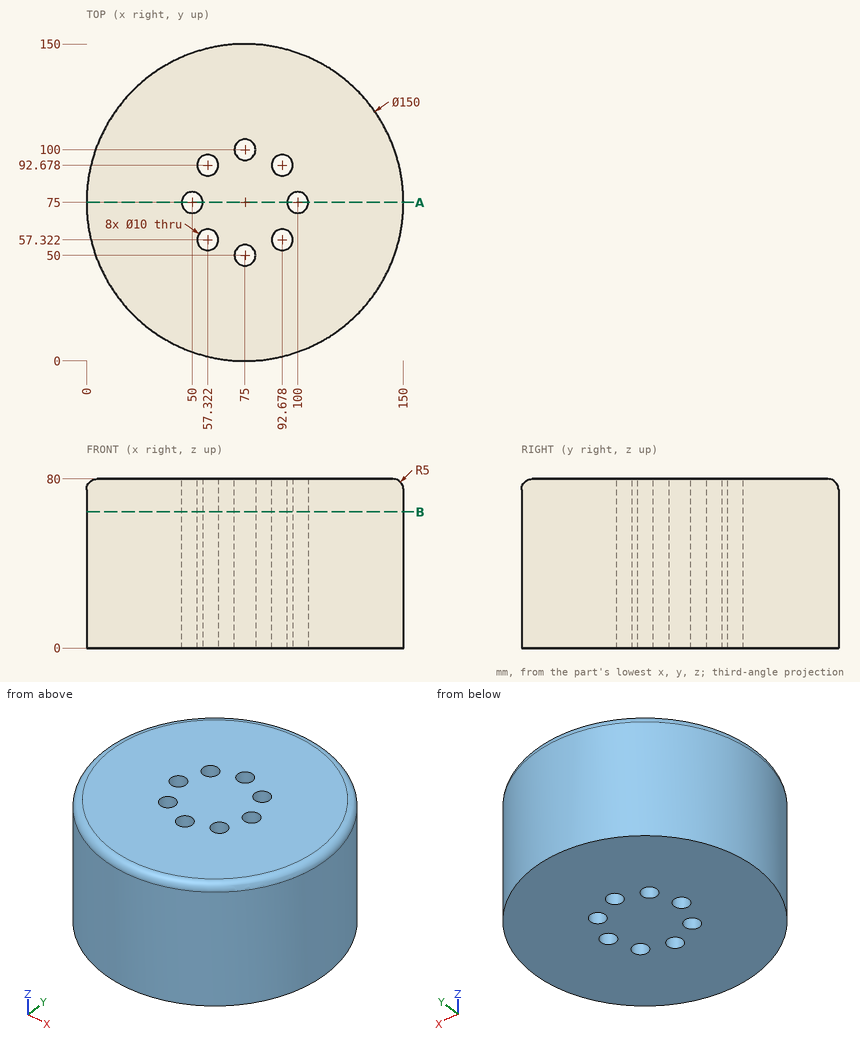
Verification items for this drawing (mm, ordinates from the low corner). Give positions to 0.01 mm unless a question says otherwise; leave off trailing zeros. Loops run counter-clockwise (first coordinate to the right, second up) from the corner with the lowest first, then second, coordinate; pieces in that order, holes last. Notation, with made-up numbers: (82, 68.25) - (119, 68.25) arc R16 cw to (119, 75.25) - close; hole circle Ø2 at (18.5, 27). An arc over 180 degrees is marked (long way). Write item = value, one per line. Start each with the question number.
Q1. Thickness scan on line 1 (X direction, y = 71, z = 29) (1 decimal); line 2 (Y direction, x = 94.5, z = 17.5); line 3 (X direction, y = 101, z = 10.5). Record the ranges inside material, lowest first.
Q2. Cross-section at A-A, the plane y = 75. Enter the section's corners in (x, z), and give its area (3 significant figures).
Q3. Depth check by flat-ended pin: P1, Ø1, axis at y = 53.5, z = 21.5, coming from the -X side; P2, Ø3, axis at y = 99.5, z = 42, coming from the +X side; P3, Ø2, axis at y = 115, z = 60.5, coming from the -X side. Enter the tip coordinate at first touch or a pass-through.
Q4. Cross-section at B-B, the plane z = 64.5. State how many separate pieces and enclosed holes the cut face has, and give its area (3 significant figures).
Answer key:
q1.line_1 = 0.1 to 47, 53 to 97, 103 to 149.9
q1.line_2 = 2.58 to 52.67, 61.98 to 88.02, 97.33 to 147.42
q1.line_3 = 4.65 to 70.1, 79.9 to 145.35
q2.outline = (0, 0) - (45, 0) - (45, 80) - (5, 80) arc R5 ccw to (0, 75) - close; (55, 0) - (95, 0) - (95, 80) - (55, 80) - close; (105, 0) - (150, 0) - (150, 75) arc R5 ccw to (145, 80) - (105, 80) - close
q2.area = 10,400 mm^2
q3.P1 = 3
q3.P2 = 146.39
q3.P3 = 10.94
q4.separate_pieces = 1
q4.enclosed_holes = 8
q4.area = 17,000 mm^2
